For this review, take the finished solid that the model builds, in its own axes (mm). Face numbers are marked on the shaded views. A direction names the side the tool comes from. Give positions to 0.01 mm unless a question says otherwise; leave off trailing zeros. Order: outer loops, then holes, each group sorted by start corner. A loop starts at its lowest first (then second) coordinate and runs counter-clockwise, first axis right, second up. Notation, with made-up numbers: (-21, 51) - (3, 51) arc R18 cw to (3, 62) - close; hole circle Ø10 at (-29, 83). An arc over 180 degrees is marked (long way). Use a Markdown table: item, result. Add a question column.
1) Mouldability with a two-part tool opening along X and no side actions: class the marked faces 1, 2, 3 and 4 as released by +X, released by -X, zero draft, split by the parting line, or undercut.
2) We need section A-A on x = 24.5. Write out the cut boundary in (y, z), then the cut area to 3 significant figures.
3) Clearance check with flat-ended pins moving along their axes: P1, Ø5, axis at y = 13, z = 5, coming from the +X side; P2, Ø1, axis at y = -10, z = 5, coming from the +X side; P3, Ø8, axis at x = -13, z = 4, coming from the +Y side. State where each tip first meets the part, or that it passes through.
4) We need section B-B on z = 6. Give the number of separate pieces and of enclosed holes in the cut face, then the cut area to 3 significant figures.
5) Machinability: for the marked faces 5, 6, 7, 8 and 9, which of the approach directions +Z, -Z, +X, -X, +Y, -Y give a long, thin tool a straight path to every point of the face, cutting with its end or side? Answer none if there is none.
6) Wall thickness on L1, parallel to Y at x = 0, z = -3; L2, parallel to Y at x = 54.5, z = 1.75; L3, parallel to Y at x = -51, z = 8.5: over which ranges is each line inside the solid? List them lowest first.
```python
from build123d import *

# Parameters (mm, degrees)
SKETCH1_W                   = 120.65
SKETCH1_H                   = 38.1
BOSS_EXTRUDE1_DEPTH         = 12.7
SKETCH2_R                   = 14.351
CUT_EXTRUDE1_DEPTH          = 12.7
F_8_32_TAPPED_HOLE1_D       = 3.4544
F_8_32_TAPPED_HOLE1_DEPTH   = 12.7
F_8_32_TAPPED_HOLE1_TIP     = 1.037806461
CUT_EXTRUDE2_REACH          = 70.17
SKETCH7_R                   = 4.7625
FILLET1_R                   = 12.7
SKETCH12_W                  = 38.1
SKETCH12_H                  = 12.827
SKETCH12_H_2                = 9.652
SKETCH12_H_3                = 6.35
CUT_EXTRUDE6_DEPTH          = 69.170141008
SKETCH13_R                  = 3.7465
CUT_EXTRUDE7_DEPTH          = 73.470722537
F_1_4_CLEARANCE_HOLE1_D     = 6.7564
F_1_4_CLEARANCE_HOLE1_DEPTH = 19.05
F_1_4_CLEARANCE_HOLE1_TIP   = 2.029827343
CHAMFER1_SIZE               = 2.54
FILLET2_R                   = 25.4
FILLET3_R                   = 12.7
FILLET4_R                   = 40.64
FILLET5_R                   = 12.7
FILLET6_R                   = 4.7625


# Some blends are built 0.0001 mm under size
with BuildPart() as part:
    # Sketch1 → Boss-Extrude1 (new, symmetric)
    with BuildSketch(Plane.XY):
        Rectangle(SKETCH1_W, SKETCH1_H)
    extrude(amount=BOSS_EXTRUDE1_DEPTH, both=True)

    # Sketch2 → Cut-Extrude1 (cut)
    with BuildSketch(Plane(origin=(0, 0, -12.7), x_dir=(-1, 0, 0), z_dir=(0, 0, -1))):
        Circle(SKETCH2_R)
    extrude(amount=-CUT_EXTRUDE1_DEPTH, mode=Mode.SUBTRACT)

    # #8-32 Tapped Hole1
    with Locations(Plane.XY.offset(12.7)):
        with Locations((9.525, 0), (-9.525, 0)):
            Hole(F_8_32_TAPPED_HOLE1_D / 2, depth=F_8_32_TAPPED_HOLE1_DEPTH)
            with Locations((0, 0, -(F_8_32_TAPPED_HOLE1_DEPTH + F_8_32_TAPPED_HOLE1_TIP / 2))):  # 118° drill point
                Cone(0, F_8_32_TAPPED_HOLE1_D / 2, F_8_32_TAPPED_HOLE1_TIP, mode=Mode.SUBTRACT)

    # Sketch7 → Cut-Extrude2 (cut, up to next)
    with BuildSketch(Plane.XY.offset(12.7), mode=Mode.PRIVATE) as cut_extrude2_sk1:
        Circle(SKETCH7_R)
    cut_extrude2_tool1 = extrude(cut_extrude2_sk1.sketch, amount=-CUT_EXTRUDE2_REACH, mode=Mode.PRIVATE) & part.part
    add(cut_extrude2_tool1.solids().sort_by_distance((0, 0, 12.7))[0], mode=Mode.SUBTRACT)

    # Fillet1
    fillet1_edges = [part.edges().sort_by_distance(p)[0] for p in [
        (-60.325, 0, 12.7),
        (-60.325, 0, -12.7),
        (60.325, 0, 12.7),
        (60.325, 0, -12.7),
    ]]
    fillet(fillet1_edges, radius=FILLET1_R - 0.0001)  # a hair under: the kernel refuses the full size

    # Sketch12 → Cut-Extrude6 (cut, through all)
    with BuildSketch(Plane.XY.offset(12.7)):
        with Locations((-41.275, 12.6365)):
            Rectangle(SKETCH12_W, SKETCH12_H)
        with Locations((41.275, 0)):
            Rectangle(SKETCH12_W, SKETCH12_H_2)
        with Locations((-41.275, -12.6365)):
            Rectangle(SKETCH12_W, SKETCH12_H)
        with Locations((41.275, 15.875)):
            Rectangle(SKETCH12_W, SKETCH12_H_3)
        with Locations((41.275, -15.875)):
            Rectangle(SKETCH12_W, SKETCH12_H_3)
    extrude(amount=-CUT_EXTRUDE6_DEPTH, mode=Mode.SUBTRACT)

    # Sketch13 → Cut-Extrude7 (cut, through all)
    with BuildSketch(Plane(origin=(0, 19.05, 0), x_dir=(1, 0, 0), z_dir=(0, 1, 0))):
        with Locations(Location((47.625, 0, 0), (0, 0, 270))):
            Circle(SKETCH13_R)
    extrude(amount=-CUT_EXTRUDE7_DEPTH, mode=Mode.SUBTRACT)

    # 1/4 Clearance Hole1
    with Locations(Plane(origin=(0, 9.525, -30.597499938), x_dir=(0, 0, 1), z_dir=(0, 1, 0))):
        with Locations((30.597499938, -47.625), (62.347499938, -47.625), (81.397499938, -47.625), (196.332499938, -47.625)):
            Hole(F_1_4_CLEARANCE_HOLE1_D / 2, depth=F_1_4_CLEARANCE_HOLE1_DEPTH)
            with Locations((0, 0, -(F_1_4_CLEARANCE_HOLE1_DEPTH + F_1_4_CLEARANCE_HOLE1_TIP / 2))):  # 118° drill point
                Cone(0, F_1_4_CLEARANCE_HOLE1_D / 2, F_1_4_CLEARANCE_HOLE1_TIP, mode=Mode.SUBTRACT)

    # Chamfer1
    chamfer1_edges = [part.edges().sort_by_distance(p)[0] for p in [
        (-4.7625, 0, 0),
    ]]
    chamfer(chamfer1_edges, length=CHAMFER1_SIZE)

    # Fillet2
    # the kernel refuses this fillet: 25.4 mm, written as the material it takes off along each edge
    with BuildSketch(Plane(origin=(-22.225, -19.05, 67.874703839), x_dir=(0, 1, 0), z_dir=(0, 0, -1))) as fillet2_piece_1:
        with BuildLine():
            CenterArc((25.4, 22.069881536), FILLET2_R, 180, 60.330249663)
            Line((0, 22.069881536), (-0.508, 22.069881536))
            Line((-0.508, 22.069881536), (-0.508, 0))
            Line((-0.508, 0), (0, -0.508))
            ThreePointArc((0, -0.508), (6.4135, -0.508), (12.57554, -0.441397631))
            Line((12.57554, -0.441397631), (12.827, 0))
        make_face()
    extrude(amount=135.749407679, mode=Mode.SUBTRACT)
    with BuildSketch(Plane(origin=(-22.225, 19.05, 67.874703839), x_dir=(0, -1, 0), z_dir=(0, 0, -1))) as fillet2_piece_2:
        with BuildLine():
            CenterArc((25.4, -22.069881536), FILLET2_R, 119.669750337, 60.330249663)
            Line((0, -22.069881536), (-0.508, -22.069881536))
            Line((-0.508, -22.069881536), (-0.508, 0))
            Line((-0.508, 0), (0, 0.508))
            ThreePointArc((0, 0.508), (6.4135, 0.508), (12.57554, 0.441397631))
            Line((12.57554, 0.441397631), (12.827, 0))
        make_face()
    extrude(amount=135.749407679, mode=Mode.SUBTRACT)

    # Fillet3
    fillet3_edges = [part.edges().sort_by_distance(p)[0] for p in [
        (-22.225, 6.223, 0),
        (-22.225, -6.223, 0),
    ]]
    fillet(fillet3_edges, radius=FILLET3_R)

    # Fillet4
    # the kernel refuses this fillet: 40.64 mm, written as the material it takes off along each edge
    with BuildSketch(Plane(origin=(22.225, -19.05, 67.232415818), x_dir=(-1, 0, 0), z_dir=(0, 0, -1))) as fillet4_piece_1:
        with BuildLine():
            CenterArc((21.812966327, 40.64), FILLET4_R, 237.538255033, 32.461744967)
            Line((0, 6.35), (-0.436259327, 5.6642))
            ThreePointArc((-0.436259327, 5.6642), (-0.8128, 3.175), (-0.8128, 0))
            Line((-0.8128, 0), (0, -0.8128))
            Line((0, -0.8128), (21.812966327, -0.8128))
            Line((21.812966327, -0.8128), (21.812966327, 0))
        make_face()
    extrude(amount=134.464831637, mode=Mode.SUBTRACT)
    with BuildSketch(Plane(origin=(22.225, 19.05, 67.232415818), x_dir=(-1, 0, 0), z_dir=(0, 0, -1))) as fillet4_piece_2:
        with BuildLine():
            CenterArc((21.812966327, -40.64), FILLET4_R, 90, 32.461744967)
            Line((0, -6.35), (-0.436259327, -5.6642))
            ThreePointArc((-0.436259327, -5.6642), (-0.8128, -3.175), (-0.8128, 0))
            Line((-0.8128, 0), (0, 0.8128))
            Line((0, 0.8128), (21.812966327, 0.8128))
            Line((21.812966327, 0.8128), (21.812966327, 0))
        make_face()
    extrude(amount=134.464831637, mode=Mode.SUBTRACT)

    # Fillet5
    fillet5_edges = [part.edges().sort_by_distance(p)[0] for p in [
        (22.225, 12.7, 0),
        (22.225, -12.7, 0),
    ]]
    fillet(fillet5_edges, radius=FILLET5_R)

    # Fillet6
    fillet6_edges = [part.edges().sort_by_distance(p)[0] for p in [
        (22.225, -4.826, 0),
        (22.225, 4.826, 0),
    ]]
    fillet(fillet6_edges, radius=FILLET6_R)


solid = part.part
```
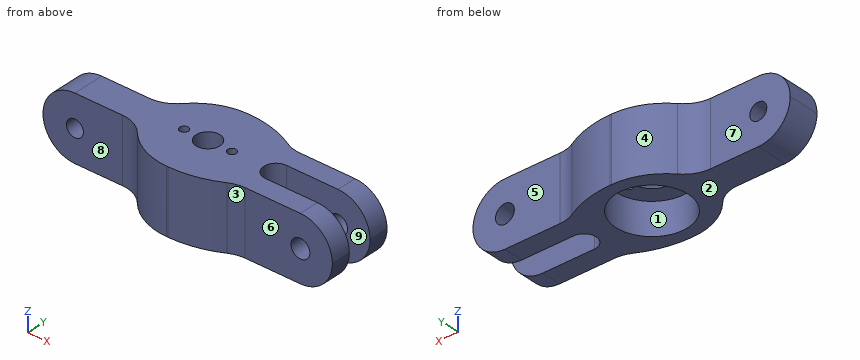
Checked values:
| question | item | result |
|---|---|---|
| 1 | face 1 | undercut |
| 1 | face 2 | zero draft |
| 1 | face 3 | released by +X |
| 1 | face 4 | released by -X |
| 2 | outline | (-12.75, -12.7) - (-4.12, -12.7) - (-4.12, 12.7) - (-12.75, 12.7) - close; (4.12, -12.7) - (12.75, -12.7) - (12.75, 12.7) - (4.12, 12.7) - close |
| 2 | area | 438 mm² |
| 3 | P1 | x = 60.07 |
| 3 | P2 | x = 59.5 |
| 3 | P3 | y = 17.46 |
| 4 | separate pieces | 1 |
| 4 | enclosed holes | 3 |
| 4 | area | 2,400 mm² |
| 5 | face 5 | +Z, -Z, +X, +Y |
| 5 | face 6 | +Z, -Z, +X, -Y |
| 5 | face 7 | +Z, -Z, -X, +Y |
| 5 | face 8 | +Z, -Z, -X, -Y |
| 5 | face 9 | +Z, -Z, +X |
| 6 | L1 | -19.05 to -14.35, 14.35 to 19.05 |
| 6 | L2 | -12.7 to -4.83, 4.83 to 12.7 |
| 6 | L3 | -6.22 to 6.22 |
